from build123d import *

# Parameters (mm, degrees)
SKETCH_1_R          = 35
SKETCH_1_R_2        = 1.6
SKETCH_1_R_3        = 1.35
SKETCH_1_R_4        = 12
EXTRUDE_1_DEPTH     = 3
CUT_EXTRUDE_1_DEPTH = 3


with BuildPart() as part:
    # 草图1 → 凸台-拉伸1 (new body)
    with BuildSketch(Plane.XY):
        Circle(SKETCH_1_R)
        with Locations((-22.627416998, 22.627416998)):
            Circle(SKETCH_1_R_2, mode=Mode.SUBTRACT)
        with Locations((0, 32)):
            Circle(SKETCH_1_R_2, mode=Mode.SUBTRACT)
        with Locations((22.627416998, 22.627416998)):
            Circle(SKETCH_1_R_2, mode=Mode.SUBTRACT)
        with Locations((32, 0)):
            Circle(SKETCH_1_R_2, mode=Mode.SUBTRACT)
        with Locations((22.627416998, -22.627416998)):
            Circle(SKETCH_1_R_2, mode=Mode.SUBTRACT)
        with Locations((0, -32)):
            Circle(SKETCH_1_R_2, mode=Mode.SUBTRACT)
        with Locations((-22.627416998, -22.627416998)):
            Circle(SKETCH_1_R_2, mode=Mode.SUBTRACT)
        with Locations((-32, 0)):
            Circle(SKETCH_1_R_2, mode=Mode.SUBTRACT)
        with Locations((-13.435028843, 13.435028843)):
            Circle(SKETCH_1_R_3, mode=Mode.SUBTRACT)
        with Locations((0, 19)):
            Circle(SKETCH_1_R_3, mode=Mode.SUBTRACT)
        with Locations((13.435028843, 13.435028843)):
            Circle(SKETCH_1_R_3, mode=Mode.SUBTRACT)
        with Locations((19, 0)):
            Circle(SKETCH_1_R_3, mode=Mode.SUBTRACT)
        with Locations((13.435028843, -13.435028843)):
            Circle(SKETCH_1_R_3, mode=Mode.SUBTRACT)
        with Locations((0, -19)):
            Circle(SKETCH_1_R_3, mode=Mode.SUBTRACT)
        with Locations((-13.435028843, -13.435028843)):
            Circle(SKETCH_1_R_3, mode=Mode.SUBTRACT)
        with Locations((-19, 0)):
            Circle(SKETCH_1_R_3, mode=Mode.SUBTRACT)
        Circle(SKETCH_1_R_4, mode=Mode.SUBTRACT)
    extrude(amount=EXTRUDE_1_DEPTH)

    # 草图2 → 切除-拉伸1 (cut)
    with BuildSketch(Plane.XY.offset(3)):
        with BuildLine():
            Line((4.026410343, 28.649398244), (3.188856349, 22.689891917))
            ThreePointArc((3.188856349, 22.689891917), (3.521253388, 21.278568437), (4.719880097, 20.462715652))
            ThreePointArc((4.719880097, 20.462715652), (8.03635208, 19.401470183), (11.131865777, 17.806784222))
            ThreePointArc((11.131865777, 17.806784222), (12.556317887, 17.536122185), (13.78931449, 18.299038387))
            Line((13.78931449, 18.299038387), (17.411081718, 23.105285833))
            ThreePointArc((17.411081718, 23.105285833), (17.783563729, 24.655431386), (16.904418332, 25.985392836))
            ThreePointArc((16.904418332, 25.985392836), (11.863186403, 28.640265508), (6.421218651, 30.327676321))
            ThreePointArc((6.421218651, 30.327676321), (4.85914422, 30.008901233), (4.026410343, 28.649398244))
        make_face()
        with BuildLine():
            Line((23.105285833, 17.411081718), (18.299038387, 13.78931449))
            ThreePointArc((18.299038387, 13.78931449), (17.536122185, 12.556317887), (17.806784222, 11.131865777))
            ThreePointArc((17.806784222, 11.131865777), (19.401470183, 8.03635208), (20.462715652, 4.719880097))
            ThreePointArc((20.462715652, 4.719880097), (21.278568437, 3.521253388), (22.689891917, 3.188856349))
            Line((22.689891917, 3.188856349), (28.649398244, 4.026410343))
            ThreePointArc((28.649398244, 4.026410343), (30.008901233, 4.85914422), (30.327676321, 6.421218651))
            ThreePointArc((30.327676321, 6.421218651), (28.640265508, 11.863186403), (25.985392836, 16.904418332))
            ThreePointArc((25.985392836, 16.904418332), (24.655431386, 17.783563729), (23.105285833, 17.411081718))
        make_face()
        with BuildLine():
            Line((28.649398244, -4.026410343), (22.689891917, -3.188856349))
            ThreePointArc((22.689891917, -3.188856349), (21.278568437, -3.521253388), (20.462715652, -4.719880097))
            ThreePointArc((20.462715652, -4.719880097), (19.401470183, -8.03635208), (17.806784222, -11.131865777))
            ThreePointArc((17.806784222, -11.131865777), (17.536122185, -12.556317887), (18.299038387, -13.78931449))
            Line((18.299038387, -13.78931449), (23.105285833, -17.411081718))
            ThreePointArc((23.105285833, -17.411081718), (24.655431386, -17.783563729), (25.985392836, -16.904418332))
            ThreePointArc((25.985392836, -16.904418332), (28.640265508, -11.863186403), (30.327676321, -6.421218651))
            ThreePointArc((30.327676321, -6.421218651), (30.008901233, -4.85914422), (28.649398244, -4.026410343))
        make_face()
        with BuildLine():
            Line((17.411081718, -23.105285833), (13.78931449, -18.299038387))
            ThreePointArc((13.78931449, -18.299038387), (12.556317887, -17.536122185), (11.131865777, -17.806784222))
            ThreePointArc((11.131865777, -17.806784222), (8.03635208, -19.401470183), (4.719880097, -20.462715652))
            ThreePointArc((4.719880097, -20.462715652), (3.521253388, -21.278568437), (3.188856349, -22.689891917))
            Line((3.188856349, -22.689891917), (4.026410343, -28.649398244))
            ThreePointArc((4.026410343, -28.649398244), (4.85914422, -30.008901233), (6.421218651, -30.327676321))
            ThreePointArc((6.421218651, -30.327676321), (11.863186403, -28.640265508), (16.904418332, -25.985392836))
            ThreePointArc((16.904418332, -25.985392836), (17.783563729, -24.655431386), (17.411081718, -23.105285833))
        make_face()
        with BuildLine():
            Line((-4.026410343, -28.649398244), (-3.188856349, -22.689891917))
            ThreePointArc((-3.188856349, -22.689891917), (-3.521253388, -21.278568437), (-4.719880097, -20.462715652))
            ThreePointArc((-4.719880097, -20.462715652), (-8.03635208, -19.401470183), (-11.131865777, -17.806784222))
            ThreePointArc((-11.131865777, -17.806784222), (-12.556317887, -17.536122185), (-13.78931449, -18.299038387))
            Line((-13.78931449, -18.299038387), (-17.411081718, -23.105285833))
            ThreePointArc((-17.411081718, -23.105285833), (-17.783563729, -24.655431386), (-16.904418332, -25.985392836))
            ThreePointArc((-16.904418332, -25.985392836), (-11.863186403, -28.640265508), (-6.421218651, -30.327676321))
            ThreePointArc((-6.421218651, -30.327676321), (-4.85914422, -30.008901233), (-4.026410343, -28.649398244))
        make_face()
        with BuildLine():
            Line((-23.105285833, -17.411081718), (-18.299038387, -13.78931449))
            ThreePointArc((-18.299038387, -13.78931449), (-17.536122185, -12.556317887), (-17.806784222, -11.131865777))
            ThreePointArc((-17.806784222, -11.131865777), (-19.401470183, -8.03635208), (-20.462715652, -4.719880097))
            ThreePointArc((-20.462715652, -4.719880097), (-21.278568437, -3.521253388), (-22.689891917, -3.188856349))
            Line((-22.689891917, -3.188856349), (-28.649398244, -4.026410343))
            ThreePointArc((-28.649398244, -4.026410343), (-30.008901233, -4.85914422), (-30.327676321, -6.421218651))
            ThreePointArc((-30.327676321, -6.421218651), (-28.640265508, -11.863186403), (-25.985392836, -16.904418332))
            ThreePointArc((-25.985392836, -16.904418332), (-24.655431386, -17.783563729), (-23.105285833, -17.411081718))
        make_face()
        with BuildLine():
            Line((-28.649398244, 4.026410343), (-22.689891917, 3.188856349))
            ThreePointArc((-22.689891917, 3.188856349), (-21.278568437, 3.521253388), (-20.462715652, 4.719880097))
            ThreePointArc((-20.462715652, 4.719880097), (-19.401470183, 8.03635208), (-17.806784222, 11.131865777))
            ThreePointArc((-17.806784222, 11.131865777), (-17.536122185, 12.556317887), (-18.299038387, 13.78931449))
            Line((-18.299038387, 13.78931449), (-23.105285833, 17.411081718))
            ThreePointArc((-23.105285833, 17.411081718), (-24.655431386, 17.783563729), (-25.985392836, 16.904418332))
            ThreePointArc((-25.985392836, 16.904418332), (-28.640265508, 11.863186403), (-30.327676321, 6.421218651))
            ThreePointArc((-30.327676321, 6.421218651), (-30.008901233, 4.85914422), (-28.649398244, 4.026410343))
        make_face()
        with BuildLine():
            Line((-17.411081718, 23.105285833), (-13.78931449, 18.299038387))
            ThreePointArc((-13.78931449, 18.299038387), (-12.556317887, 17.536122185), (-11.131865777, 17.806784222))
            ThreePointArc((-11.131865777, 17.806784222), (-8.03635208, 19.401470183), (-4.719880097, 20.462715652))
            ThreePointArc((-4.719880097, 20.462715652), (-3.521253388, 21.278568437), (-3.188856349, 22.689891917))
            Line((-3.188856349, 22.689891917), (-4.026410343, 28.649398244))
            ThreePointArc((-4.026410343, 28.649398244), (-4.85914422, 30.008901233), (-6.421218651, 30.327676321))
            ThreePointArc((-6.421218651, 30.327676321), (-11.863186403, 28.640265508), (-16.904418332, 25.985392836))
            ThreePointArc((-16.904418332, 25.985392836), (-17.783563729, 24.655431386), (-17.411081718, 23.105285833))
        make_face()
    extrude(amount=-CUT_EXTRUDE_1_DEPTH, mode=Mode.SUBTRACT)


solid = part.part
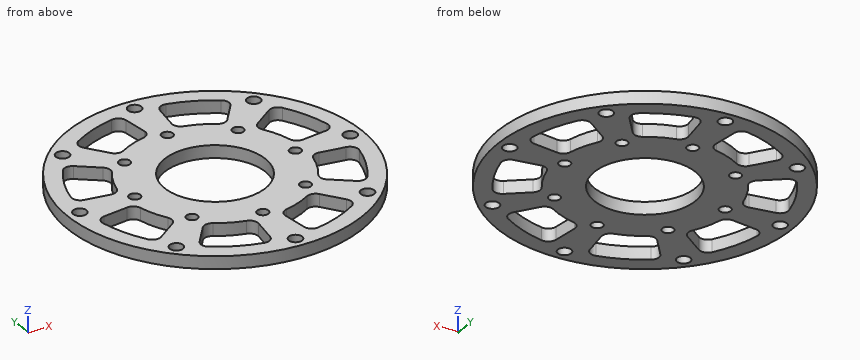
Model file for the job. Use its own axes, mm. Give positions to 0.01 mm unless a question says otherwise; leave off trailing zeros. Write each loop counter-clockwise with the first axis right and the second up, starting at its lowest first coordinate (ties: lowest second). Pieces come first, ordered by that corner, then holes. Notation, with made-up numbers: M -14,48 L 15,48 A16 cw 15,58 Z; hole C 64,39.5 d9. An arc over 180 degrees is marked long. One line per item, written item: value. Start each with the question number.
Q1. Saw through at A-A, the plane y = -32. Write the cut outline in (x, z).
Q2. Drop flat-ended pins along their axis: pin 1 Ø3 at (x, y) = (-13.44, -13.44) entering from -Z; pin 2 Ø1 at (x, z) = (-15.5, 1) entering from +Y; pin 3 Ø1.5 at (x, z) = (-18.5, 0.5) entering from -Y. Give the stop position or say it passes through.
Q3. Saw through at C-C, the plane z = 0.8. State how many separate pieces and enclosed holes the cut face has, plus the area to 3 significant figures.
Q4. Probe probe 1 along Y at (x, z) = (0, 1.25); probe 2 along Y at (x, z) = (-17, 0.9); probe 3 along X at (y, z) = (12.5, 2.1). List the from-to ranges inside material, lowest first. Write a range as [from, to].
Output values:
1. outline: M -14.18,0 L -1.6,0 L -1.6,3 L -14.18,3 Z; M 1.6,0 L 14.18,0 L 14.18,3 L 1.6,3 Z
2. pin 1: stops at z = 0
2. pin 2: stops at y = 31.62
2. pin 3: stops at y = -30.17
3. separate pieces: 1
3. enclosed holes: 25
3. area: 2,260 mm²
4. probe 1: y = [-35, -33.6], [-30.4, -20.35], [-17.65, -12], [12, 17.65], [20.35, 30.4], [33.6, 35]
4. probe 2: y = [-30.59, -25.92], [-22.56, 22.56], [25.92, 30.59]
4. probe 3: x = [-32.69, -28.37], [-17.53, -14.41], [-12.46, 12.46], [14.41, 17.53], [28.37, 32.69]
